```python
from build123d import *

# Parameters (mm, degrees)
CYLINDER004_R          = 18
CYLINDER004_DEPTH      = 10
CYLINDER002_R          = 1.7
CYLINDER002_DEPTH      = 10
CYLINDER001_R          = 1.7
CYLINDER001_DEPTH      = 10
CYLINDER003_R          = 1.7
CYLINDER003_DEPTH      = 10
CYLINDER_R             = 1.7
CYLINDER_DEPTH         = 10
BOX_W                  = 37
BOX_H                  = 37
BOX_DEPTH              = 3
CYLINDER005_R          = 20
CYLINDER005_DEPTH      = 10
CYLINDER006_R          = 1.7
CYLINDER006_DEPTH      = 10
CYLINDER007_R          = 1.7
CYLINDER007_DEPTH      = 10
BOX004_W               = 20
BOX004_H               = 20
BOX004_DEPTH           = 10
BOX004_PITCH_ANGLE     = -44.999934
BOX003_W               = 20
BOX003_H               = 20
BOX003_DEPTH           = 10
BOX003_PITCH_ANGLE     = 44.999934
BOX002_W               = 56
BOX002_H               = 20
BOX002_DEPTH           = 10
BOX001_W               = 40
BOX001_H               = 40
BOX001_DEPTH           = 10
BOX001_PLACEMENT_ANGLE = 44.999934


with BuildPart() as obj1:
    # Cylinder004 → Cylinder004 (new body)
    with BuildSketch(Plane.XY):
        Circle(CYLINDER004_R)
    extrude(amount=CYLINDER004_DEPTH)


with BuildPart() as cylinder002:
    # Cylinder002 → Cylinder002 (new body)
    with BuildSketch(Plane(origin=(31, 31, 0), x_dir=(1, 0, 0), z_dir=(0, 0, 1))):
        Circle(CYLINDER002_R)
    extrude(amount=CYLINDER002_DEPTH)


with BuildPart() as cylinder001:
    # Cylinder001 → Cylinder001 (new body)
    with BuildSketch(Plane(origin=(31, 0, 0), x_dir=(1, 0, 0), z_dir=(0, 0, 1))):
        Circle(CYLINDER001_R)
    extrude(amount=CYLINDER001_DEPTH)


with BuildPart() as cylinder003:
    # Cylinder003 → Cylinder003 (new body)
    with BuildSketch(Plane(origin=(0, 31, 0), x_dir=(1, 0, 0), z_dir=(0, 0, 1))):
        Circle(CYLINDER003_R)
    extrude(amount=CYLINDER003_DEPTH)


with BuildPart() as obj2:
    # Cylinder → Cylinder (new body)
    with BuildSketch(Plane.XY):
        Circle(CYLINDER_R)
    extrude(amount=CYLINDER_DEPTH)

    # Fusion: union Cylinder002, Cylinder001, Cylinder003
    add(cylinder002.part)
    add(cylinder001.part)
    add(cylinder003.part)


with BuildPart() as obj2_1:
    # Fusion placement: moved
    add(obj2.part.moved(Location((-15.5, -15.5, 0))))


with BuildPart() as obj3:
    # Box → Box (new body)
    with BuildSketch(Plane(origin=(-18.5, -18.5, 7), x_dir=(1, 0, 0), z_dir=(0, 0, 1))):
        with Locations((18.5, 18.5)):
            Rectangle(BOX_W, BOX_H)
    extrude(amount=BOX_DEPTH)

    # Cut001: cut obj2
    add(obj2_1.part, mode=Mode.SUBTRACT)


with BuildPart() as basis:
    # Cylinder005 → Cylinder005 (new body)
    with BuildSketch(Plane.XY):
        Circle(CYLINDER005_R)
    extrude(amount=CYLINDER005_DEPTH)


with BuildPart() as cylinder006:
    # Cylinder006 → Cylinder006 (new body)
    with BuildSketch(Plane(origin=(-24, 0, 0), x_dir=(1, 0, 0), z_dir=(0, 0, 1))):
        Circle(CYLINDER006_R)
    extrude(amount=CYLINDER006_DEPTH)


with BuildPart() as obj4:
    # Cylinder007 → Cylinder007 (new body)
    with BuildSketch(Plane(origin=(24, 0, 0), x_dir=(1, 0, 0), z_dir=(0, 0, 1))):
        Circle(CYLINDER007_R)
    extrude(amount=CYLINDER007_DEPTH)

    # Fusion001: union Cylinder006
    add(cylinder006.part)


with BuildPart() as box004:
    # Box004 → Box004 (new body)
    with BuildSketch(Plane.XY):
        with Locations((10, 10)):
            Rectangle(BOX004_W, BOX004_H)
    extrude(amount=BOX004_DEPTH)


with BuildPart() as box004_1:
    # Box004 pitch: moved
    add(box004.part.rotate(Axis((0, 0, 0), (0, 1, 0)), BOX004_PITCH_ANGLE))


with BuildPart() as box004_2:
    # Box004 placement: moved
    add(box004_1.part.moved(Location((-30, -10, 0))))


with BuildPart() as obj5:
    # Box003 → Box003 (new body)
    with BuildSketch(Plane.XY):
        with Locations((10, 10)):
            Rectangle(BOX003_W, BOX003_H)
    extrude(amount=BOX003_DEPTH)


with BuildPart() as obj5_1:
    # Box003 pitch: moved
    add(obj5.part.rotate(Axis((0, 0, 0), (0, 1, 0)), BOX003_PITCH_ANGLE))


with BuildPart() as obj5_2:
    # Box003 placement: moved
    add(obj5_1.part.moved(Location((15, -10, 15))))

    # Fusion002: union Box004
    add(box004_2.part)


with BuildPart() as obj6:
    # Box002 → Box002 (new body)
    with BuildSketch(Plane(origin=(-28, -10, 0), x_dir=(1, 0, 0), z_dir=(0, 0, 1))):
        with Locations((28, 10)):
            Rectangle(BOX002_W, BOX002_H)
    extrude(amount=BOX002_DEPTH)

    # Cut: cut obj5
    add(obj5_2.part, mode=Mode.SUBTRACT)


with BuildPart() as obj7:
    # Box001 → Box001 (new body)
    with BuildSketch(Plane.XY):
        with Locations((20, 20)):
            Rectangle(BOX001_W, BOX001_H)
    extrude(amount=BOX001_DEPTH)


with BuildPart() as obj7_1:
    # Box001 placement: moved
    add(obj7.part.moved(Location((0, -28, 0))).rotate(Axis((0, -28, 0), (0, 0, 1)), BOX001_PLACEMENT_ANGLE))

    # Common: intersect obj6
    add(obj6.part, mode=Mode.INTERSECT)

    # Cut002: cut obj4
    add(obj4.part, mode=Mode.SUBTRACT)

    # Fusion003: union obj3, Basis
    add(obj3.part)
    add(basis.part)

    # Cut003: cut obj1
    add(obj1.part, mode=Mode.SUBTRACT)


solid = obj7_1.part
```
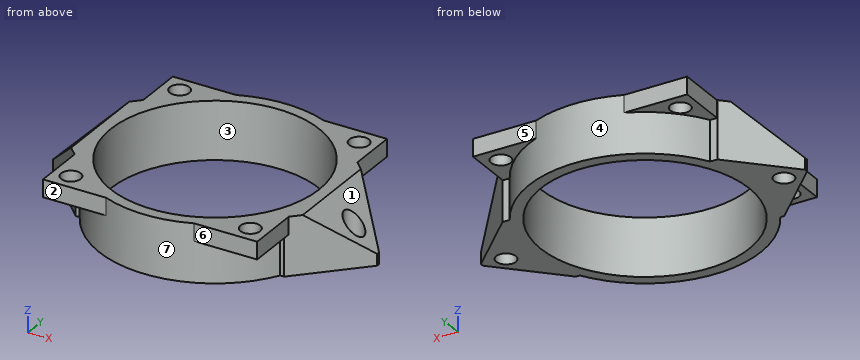
Model file for the job. Use its own axes, mm. Face numbers are marked on the shaded views. A direction names the side the tool comes from. Round coordinates to 2 decimals unless told otherwise and drop trailing zeros. Write each loop counter-clockwise with the first axis right and the second up, starting at its lowest first coordinate (ties: lowest second). Pieces come first, ordered by that corner, then holes. Notation, with made-up numbers: (45.25, 38) -> (78.25, 38) arc R28 ccw to (78.25, 71) -> close; hole circle Ø8 at (76, -31.75). An arc over 180 degrees is marked (long way). Answer as CSV lines item,"result".
1. Slice it at B-B, the plane y = -4. List the corners of the cut face in (x, z).
Resolved:
outline,"(-24, 0) -> (-17.55, 0) -> (-17.55, 10) -> (-20, 10) -> (-24, 6) -> close; (17.55, 0) -> (24, 0) -> (24, 6) -> (20, 10) -> (17.55, 10) -> close"
2. Slice it at D-D, the plane y = -15.5. List the corners of the cut face in (x, z), plus the area to 3 significant figures.
Resolved:
outline,"(-18.5, 7) -> (-17.2, 7) -> (-17.2, 10) -> (-18.5, 10) -> close; (-13.8, 7) -> (-12.64, 7) -> (-12.64, 0) -> (-9.15, 0) -> (-9.15, 10) -> (-13.8, 10) -> close; (9.15, 0) -> (12.64, 0) -> (12.64, 7) -> (13.8, 7) -> (13.8, 10) -> (9.15, 10) -> close; (17.2, 7) -> (18.5, 7) -> (18.5, 10) -> (17.2, 10) -> close"
area,"84.5 mm²"
3. Slice it at C-C, the plane z = 8.5. List the corners of the cut face in (x, y).
Resolved:
outline,"(-21.5, -6.5) -> (-18.5, -9.5) -> (-18.5, -18.5) -> (-7.6, -18.5) arc R20 ccw to (7.6, -18.5) -> (18.5, -18.5) -> (18.5, -9.5) -> (21.5, -6.5) -> (21.5, 7.07) -> (18.57, 10) -> (18.5, 10) -> (18.5, 18.5) -> (7.6, 18.5) arc R20 ccw to (-7.6, 18.5) -> (-18.5, 18.5) -> (-18.5, 10) -> (-18.57, 10) -> (-21.5, 7.07) -> close; hole circle Ø36 at (0, 0); hole circle Ø3.4 at (-15.5, -15.5); hole circle Ø3.4 at (-15.5, 15.5); hole circle Ø3.4 at (15.5, -15.5); hole circle Ø3.4 at (15.5, 15.5)"
4. Pin check, flat tips, straight feed: pin 1 Ø1.5 at (y, z) = (2.5, 6.5) entering from -X; pin 2 Ø1.5 at (y, z) = (15.5, 9) entering from -X; pin 3 Ø4 at (x, z) = (-19.5, 3) entering from +Y. Stop position of each tip, or through.
Resolved:
pin 1,"x = -24.25"
pin 2,"x = -18.5"
pin 3,"y = 10"
5. Tool access for the marked faces 4, 5, 6 and 7: list every direction of +Z, -Z, +X, -X, +Y, -Y with a clear straight run to the whole face (end or side of a thin tool).
Resolved:
face 4,"-Z, +Y"
face 5,"+Z, -Z, +X, +Y"
face 6,"+Z, -Z, +X, -Y"
face 7,"-Z, -Y"
6. Slice it at A-A, the plane x = 0. List the corners of the cut face in (y, z), plus the area to 3 significant figures.
Resolved:
outline,"(-20, 0) -> (-18, 0) -> (-18, 10) -> (-20, 10) -> close; (18, 0) -> (20, 0) -> (20, 10) -> (18, 10) -> close"
area,"40.0 mm²"
7. Mould opens along Y. For the marked faces 1, 2 and 3 say: +Y half, -Y half, draft (parallel to the pull), parting line (faces both ways), or undercut.
Resolved:
face 1,"draft"
face 2,"-Y half"
face 3,"undercut"
8. Drill centre lines: line 1 (X direction, y = 15.5, z = 8.1); line 2 (X direction, y = 5, z = 5.5). Where is each one in solid material? Low to high.
Resolved:
line 1,"-18.5 to -17.2, -13.8 to -9.15, 9.15 to 13.8, 17.2 to 18.5"
line 2,"-23.57 to -17.29, 17.29 to 23.57"
